The listing builds one solid part. Answer for the finished solid, in the listing's coordinates (mm). A direction names the side the tool comes from. Round coordinates to 2 decimals unless told otherwise and drop trailing zeros. Order: outer loops, then holes, each group sorted by start corner. A loop starts at its lowest first (then second) coordinate and runs counter-clockwise, first axis right, second up. Notation, with made-up numbers: M 53,2.5 L 80,2.5 A4 cw 80,6.5 Z; hole C 41,-16 d3. An arc over 180 degrees is marked long. Put each result on its own line as item: value. Start each with the question number.
1. Which of the six approach directions +Z, -Z, +X, -X, +Y, -Y give full straight-line access (tool end or side, diameter ignored) to faces 4 (the face through (25.745, -19.479, 2.348)), 5 (the face through (114, 26.433, 2)), 6 (the face through (25.4, 29, 2))?
2. The part is cut by section C-C (z = 3.1). Give the vertices of the cut face in (x, y) (3 decimals).
3. The part is cut by section A-A (x = 120.65). Give the vertices of the cut face in (y, z) (1 decimal), then the cut area to 3 significant figures.
4. The part is cut by section B-B (y = -26). Give the vertices of the cut face in (x, z), then the cut area to 3 significant figures.
5. The part is cut by section D-D (x = 45.5). Give the vertices of the cut face in (y, z).
6. Consider line 1 (Y direction, x = 120.65, z = 3.35) (3 decimals); line 2 (X direction, y = 20, z = 1.1); line 3 (Y direction, x = 37, z = 3.2). Determine where each line is inside the solid, lowest interval first.
7. Each of these flat-tipped pins is pushed along its axis until it touches: pin 1 Ø1.4 at (y, z) = (29.5, 2.5) entering from -X; pin 2 Ø2 at (y, z) = (-46, 1) entering from +X; pin 3 Ø1.4 at (x, z) = (17.5, 3) entering from +Y. Where does it stop, or does it pass through?
8. The mould has two halves that part along Y. Classify faces 1 (the face through (76.2, 29, 2)), 2 (the face through (38.555, -23.674, 2.348)), 3 (the face through (89, 31.196, 2)): +Y half, -Y half, draft (parallel to the pull), parting line (faces both ways), or undercut.
from build123d import *

# Parameters (mm, degrees)
SKETCH1_R           = 3.175
BOSS_EXTRUDE1_DEPTH = 4.7625


with BuildPart() as part:
    # Sketch1 → Boss-Extrude1 (new body)
    with BuildSketch(Plane.XY):
        with BuildLine():
            Line((50.8, 26.433162162), (76.2, 26.433162162))
            Line((76.2, 26.433162162), (76.2, 31.195662162))
            Line((76.2, 31.195662162), (101.6, 31.195662162))
            Line((101.6, 31.195662162), (101.6, 26.433162162))
            Line((101.6, 26.433162162), (127, 26.433162162))
            Line((127, 26.433162162), (127, 1.01998892))
            Line((127, 1.01998892), (28.57520326, 1.01998892))
            ThreePointArc((28.57520326, 1.01998892), (38.742465974, -24.003706053), (55.140964092, -45.46641326))
            ThreePointArc((55.140964092, -45.46641326), (55.140964092, -63.426925502), (37.180451849, -63.426925502))
            ThreePointArc((37.180451849, -63.426925502), (9.624103867, -22.201039712), (-0.05269216, 26.433162162))
            Line((-0.05269216, 26.433162162), (25.4, 26.433162162))
            Line((25.4, 26.433162162), (25.4, 31.195662162))
            Line((25.4, 31.195662162), (50.8, 31.195662162))
            Line((50.8, 31.195662162), (50.8, 26.433162162))
        make_face()
        with Locations((120.65, 19.05)):
            Circle(SKETCH1_R, mode=Mode.SUBTRACT)
        with BuildLine():
            ThreePointArc((15.995135135, 20.234189189), (12.675972973, 23.258162162), (9.652, 19.939))
            ThreePointArc((9.652, 19.939), (19.70325304, -21.526564047), (43.895465689, -56.671372149))
            ThreePointArc((43.895465689, -56.671372149), (48.405772001, -56.691733412), (48.385410738, -52.1814271))
            ThreePointArc((48.385410738, -52.1814271), (25.511627679, -18.960863581), (15.995135135, 20.234189189))
        make_face(mode=Mode.SUBTRACT)
    extrude(amount=BOSS_EXTRUDE1_DEPTH)


solid = part.part
Resolved:
1. face 4: +Z, -Z
1. face 5: +Z, -Z, +X, +Y
1. face 6: +Z, -Z, -X, +Y
2. outline: M -0.053,26.433 A127.053 ccw 37.18,-63.427 A12.7 ccw 55.141,-45.466 A101.653 cw 28.575,1.02 L 127,1.02 L 127,26.433 L 101.6,26.433 L 101.6,31.196 L 76.2,31.196 L 76.2,26.433 L 50.8,26.433 L 50.8,31.196 L 25.4,31.196 L 25.4,26.433 Z; hole M 9.652,19.939 A117.528 ccw 43.895,-56.671 A3.175 ccw long 48.385,-52.181 A111.178 cw 15.995,20.234 A3.175 ccw Z; hole C 120.65,19.05 d6.35
3. outline: M 1,0 L 15.9,0 L 15.9,4.8 L 1,4.8 Z; M 22.2,0 L 26.4,0 L 26.4,4.8 L 22.2,4.8 Z
3. area: 90.8 mm2
4. outline: M 11.27,0 L 21.82,0 L 21.82,4.76 L 11.27,4.76 Z; M 28.96,0 L 39.91,0 L 39.91,4.76 L 28.96,4.76 Z
4. area: 102 mm2
5. outline: M -67.13,0 L -57.55,0 L -57.55,4.76 L -67.13,4.76 Z; M -49.19,0 L -34.32,0 L -34.32,4.76 L -49.19,4.76 Z; M 1.02,0 L 31.2,0 L 31.2,4.76 L 1.02,4.76 Z
6. line 1: 1.02 to 15.875, 22.225 to 26.433
6. line 2: 0.11 to 9.65, 16.01 to 117.62, 123.68 to 127
6. line 3: -63.25 to -49.15, -38.84 to -20.82, 1.02 to 31.2
7. pin 1: x = 25.4
7. pin 2: x = 56.45
7. pin 3: y = 26.43
8. face 1: draft
8. face 2: undercut
8. face 3: +Y half
